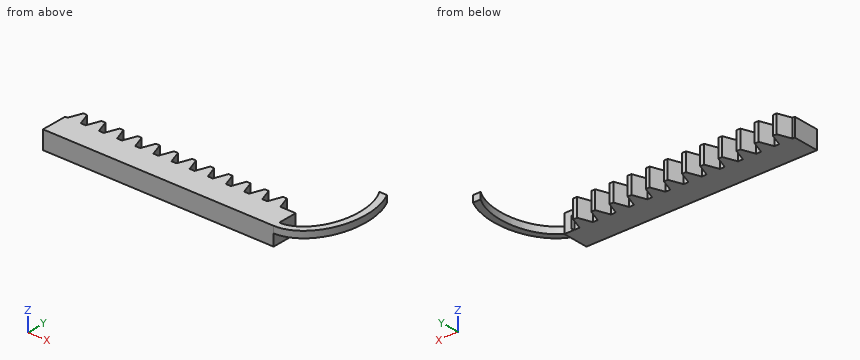
from build123d import *

# Parameters (mm, degrees)
BLANKSKE_W          = 100
BLANKSKE_H          = 11.75
BLANK_DEPTH         = 10
TOOTHCUTSIM_DEPTH   = 102.183311371
TEETHCUTS_COUNT     = 19
TEETHCUTS_PITCH     = 5.497787137
SKETCH_3_W          = 2.841503757
SKETCH_3_H          = 7.8125
EXTRUDE_1_DEPTH     = 10
EXTRUDE_2_DEPTH     = 2
SKETCH_6_W          = 102.841503757
SKETCH_6_H          = 15
CUT_EXTRUDE_2_DEPTH = 4.5
SKETCH_7_W          = 1.160244479
SKETCH_7_H          = 1.204796587
CUT_EXTRUDE_3_DEPTH = 2
SKETCH_8_W          = 16.666168626
SKETCH_8_H          = 26.64996686
CUT_EXTRUDE_5_DEPTH = 33
SKETCH_11_W         = 35.593118123
SKETCH_11_H         = 14.823069144
CUT_EXTRUDE_6_DEPTH = 2


with BuildPart() as part:
    # BlankSke → Blank (new body)
    with BuildSketch(Plane.XY):
        with Locations((50, 5.875)):
            Rectangle(BLANKSKE_W, BLANKSKE_H)
    extrude(amount=-BLANK_DEPTH)

    # TooCutSkeSim → ToothCutSim (cut, through all)
    with BuildSketch(Plane.XY):
        Polygon((0.737261897, 7.8125), (-0.737261897, 7.8125), (-2.179639538, 11.7754), (2.179639538, 11.7754), align=None)
    toothcutsim = extrude(amount=-TOOTHCUTSIM_DEPTH, mode=Mode.SUBTRACT)

    # TeethCuts: ToothCutSim ×19
    with Locations(*[(i * TEETHCUTS_PITCH, 0, 0) for i in range(1, TEETHCUTS_COUNT)]):
        add(toothcutsim, mode=Mode.SUBTRACT)

    # 草图3 → 凸台-拉伸1 (add)
    with BuildSketch(Plane.XY):
        with Locations((101.420751878, 3.90625)):
            Rectangle(SKETCH_3_W, SKETCH_3_H)
    extrude(amount=-EXTRUDE_1_DEPTH)

    # 草图5 → 凸台-拉伸2 (add)
    with BuildSketch(Plane.XY):
        with BuildLine():
            Line((102.841503757, 0), (102.841503757, 2))
            add(Edge.make_bspline(
                [(102.841503757, 2), (103.50529782, 2), (104.816875637, 2.17763142), (107.423271086, 3.255207974), (110.468253334, 6.015081397), (113.046627851, 11.280911472), (113.96899522, 17.633214309), (113.046627851, 23.985517146), (110.468253334, 29.251347221), (107.423271086, 32.011220644), (104.816875637, 33.088797198), (103.50529782, 33.266428618), (102.841503757, 33.266428618)],
                knots=[3.141592654, 3.141592654, 3.141592654, 3.141592654, 3.337942194, 3.534291735, 3.926990817, 4.319689899, 4.71238898, 5.105088062, 5.497787144, 5.890486225, 6.086835766, 6.283185307, 6.283185307, 6.283185307, 6.283185307], degree=3))
            Line((102.841503757, 33.266428618), (102.841503757, 35.266428618))
            add(Edge.make_bspline(
                [(102.841503757, 0), (115.66153943, 0), (115.66153943, 17.633214309), (115.66153943, 35.266428618), (102.841503757, 35.266428618)],
                knots=[3.141592654, 3.141592654, 3.141592654, 4.71238898, 4.71238898, 6.283185307, 6.283185307, 6.283185307], degree=2, weights=[1, 0.707106781, 1, 0.707106781, 1]))
        make_face()
    extrude(amount=-EXTRUDE_2_DEPTH)

    # 草图6 → 切除-拉伸2 (cut)
    with BuildSketch(Plane(origin=(0, 0, -10), x_dir=(-1, 0, 0), z_dir=(0, 0, -1))):
        with Locations((-51.420751879, 7.5)):
            Rectangle(SKETCH_6_W, SKETCH_6_H)
    extrude(amount=-CUT_EXTRUDE_2_DEPTH, mode=Mode.SUBTRACT)

    # 草图7 → 切除-拉伸3 (cut)
    with BuildSketch(Plane.XY):
        with Locations((99.931909363, 8.414898294)):
            Rectangle(SKETCH_7_W, SKETCH_7_H)
    extrude(amount=-CUT_EXTRUDE_3_DEPTH, mode=Mode.SUBTRACT)

    # 草图8 → 切除-拉伸5 (cut)
    with BuildSketch(Plane.ZY):
        Rectangle(SKETCH_8_W, SKETCH_8_H)
    extrude(amount=-CUT_EXTRUDE_5_DEPTH, mode=Mode.SUBTRACT)

    # 草图11 → 切除-拉伸6 (cut)
    with BuildSketch(Plane.XY):
        with Locations((104.465105415, 35.385155424)):
            Rectangle(SKETCH_11_W, SKETCH_11_H)
    extrude(amount=-CUT_EXTRUDE_6_DEPTH, mode=Mode.SUBTRACT)


solid = part.part
Verification items for the finished model (mm, model axes). Give positions to 0.01 mm unless a question says otherwise; leave off trailing zeros. Put each result on its own line as item: value. Start each with the question number.
1. Go/stop test with flat-tipped pins: pin 1 Ø0.6 at (x, z) = (57.5, -3) entering from +Y; pin 2 Ø0.7 at (x, z) = (82.5, -1.5) entering from +Y; pin 3 Ø6 at (x, y) = (93, 9.5) entering from -Z. Record where each tip stops, or that it passes through.
2. Scan lines: line 1 along X through (y, z) = (17, -0.15); line 2 along Y through (x, z) = (43.5, -0.65); line 3 along Y through (x, z) = (69, -4.35). Record each from-to range of solid material in increasing order. Write a range as [from, to].
3. Section check A-A (y = 11). Give the number of separate pieces and of enclosed holes in the cut face, and give its area (3 significant figures).
Answer list:
1. pin 1: y = 11.75
1. pin 2: y = 7.81
1. pin 3: z = -5.5
2. line 1: [113.65, 115.65]
2. line 2: [0, 7.81]
2. line 3: [0, 11.75]
3. separate pieces: 13
3. enclosed holes: 0
3. area: 117 mm2
